Build history of the part. All positions in model axes, mm. Face numbers are marked on the shaded views. A direction names the side the tool comes from. Coordinates: 2 decimals unless noted, no trailing zeros. Order: outer loops, then holes, each group sorted by start corner. A loop starts at its lowest first (then second) coordinate and runs counter-clockwise, first axis right, second up. Notation, with made-up numbers: (-24, 32.5) - (29, 32.5) arc R10 ccw to (29, 49.5) - close; hole circle Ø4 at (22, 56.25). An arc over 180 degrees is marked (long way). One line per item, written item: value.
from build123d import *

# Parameters (mm, degrees)
SKETCH1_W           = 50
SKETCH1_H           = 80
BOSS_EXTRUDE1_DEPTH = 3
SKETCH2_W           = 50
SKETCH2_H           = 3
BOSS_EXTRUDE2_DEPTH = 20
FILLET1_R           = 3
FILLET2_R           = 15
CUT_EXTRUDE1_DEPTH  = 4
CUT_EXTRUDE2_DEPTH  = 81


with BuildPart() as part:
    # Sketch1 → Boss-Extrude1 (new body)
    with BuildSketch(Plane(origin=(0, 0, 0), x_dir=(1, 0, 0), z_dir=(0, 1, 0))):
        Rectangle(SKETCH1_W, SKETCH1_H)
    extrude(amount=BOSS_EXTRUDE1_DEPTH)

    # Sketch2 → Boss-Extrude2 (add)
    with BuildSketch(Plane(origin=(0, 3, 0), x_dir=(1, 0, 0), z_dir=(0, 1, 0))):
        with Locations((0, -38.5)):
            Rectangle(SKETCH2_W, SKETCH2_H)
    extrude(amount=BOSS_EXTRUDE2_DEPTH)

    # Fillet1
    fillet1_edges = [part.edges().sort_by_distance(p)[0] for p in [
        (-25, 23, 38.5),
        (25, 23, 38.5),
    ]]
    fillet(fillet1_edges, radius=FILLET1_R)

    # Fillet2
    fillet2_edges = [part.edges().sort_by_distance(p)[0] for p in [
        (-25, 1.5, -40),
        (25, 1.5, -40),
    ]]
    fillet(fillet2_edges, radius=FILLET2_R)

    # Sketch3 → Cut-Extrude1 (cut, through all)
    with BuildSketch(Plane(origin=(0, 3, 0), x_dir=(1, 0, 0), z_dir=(0, 1, 0))):
        with BuildLine():
            Line((-12.1, 30.1), (12.1, 30.1))
            ThreePointArc((12.1, 30.1), (14.221320344, 29.221320344), (15.1, 27.1))
            Line((15.1, 27.1), (15.1, -27.1))
            ThreePointArc((15.1, -27.1), (14.221320344, -29.221320344), (12.1, -30.1))
            Line((12.1, -30.1), (-12.1, -30.1))
            ThreePointArc((-12.1, -30.1), (-14.221320344, -29.221320344), (-15.1, -27.1))
            Line((-15.1, -27.1), (-15.1, 27.1))
            ThreePointArc((-15.1, 27.1), (-14.221320344, 29.221320344), (-12.1, 30.1))
        make_face()
    extrude(amount=-CUT_EXTRUDE1_DEPTH, mode=Mode.SUBTRACT)

    # Sketch4 → Cut-Extrude2 (cut, through all)
    with BuildSketch(Plane.XY.offset(40)):
        with BuildLine():
            Line((-15, 8.5), (-15, 10))
            Line((-15, 10), (-13.5, 10))
            ThreePointArc((-13.5, 10), (-16.060660172, 11.060660172), (-15, 8.5))
        make_face()
        with BuildLine():
            Line((-13.5, 10), (-15, 10))
            Line((-15, 10), (-15, 8.5))
            ThreePointArc((-15, 8.5), (-13.939339828, 8.939339828), (-13.5, 10))
        make_face()
        with BuildLine():
            ThreePointArc((16.5, 10), (15, 11.5), (13.5, 10))
            Line((13.5, 10), (15, 10))
            Line((15, 10), (15, 8.5))
            ThreePointArc((15, 8.5), (16.060660172, 8.939339828), (16.5, 10))
        make_face()
        with BuildLine():
            Line((15, 10), (13.5, 10))
            ThreePointArc((13.5, 10), (13.939339828, 8.939339828), (15, 8.5))
            Line((15, 8.5), (15, 10))
        make_face()
    extrude(amount=-CUT_EXTRUDE2_DEPTH, mode=Mode.SUBTRACT)


solid = part.part
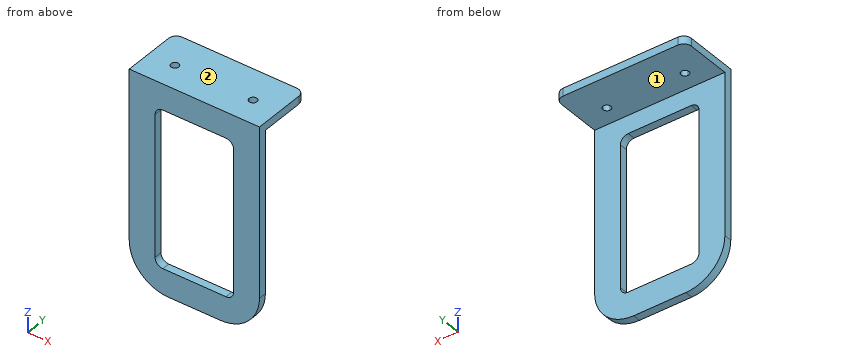
1. Flat gauge pins, fed straight in: P1, Ø1.8, axis at x = -15, y = 10, coming from the +Z side; P2, Ø10, axis at y = 4, z = 28, coming from the +X side. Where does each tip first touch, or does it go through?
Values found:
P1: passes through
P2: stops at x = 25
2. Band-saw the part on B-B, the plane x = -8.5. Give the cut face in (y, z).
Values found:
outline: (0, -40) - (3, -40) - (3, -30.1) - (0, -30.1) - close; (0, 30.1) - (3, 30.1) - (3, 37) - (23, 37) - (23, 40) - (0, 40) - close
3. Band-saw the part on A-A, the plane z = -16.5. Give the cut face in (x, y), and give its area (3 significant figures).
Values found:
outline: (-25, 0) - (-15.1, 0) - (-15.1, 3) - (-25, 3) - close; (15.1, 0) - (25, 0) - (25, 3) - (15.1, 3) - close
area: 59.4 mm2
4. Band-saw the part on C-C, the plane z = -34. Give the cut face in (x, y).
Values found:
outline: (-22, 0) - (22, 0) - (22, 3) - (-22, 3) - close
5. Band-saw the part on D-D, the plane y = 14. Give the cut face in (x, z), and give its area (3 significant figures).
Values found:
outline: (-25, 37) - (25, 37) - (25, 40) - (-25, 40) - close
area: 150 mm2
6. Probe line 1 along X through (y, z) = (10, 38); line 2 along Y through (x, z) = (-15, 38); line 3 along X through (y, z) = (2.25, -23). List the from-to ranges inside material, lowest first.
Values found:
line 1: x = -25 to -16.5, -13.5 to 13.5, 16.5 to 25
line 2: y = 0 to 8.5, 11.5 to 23
line 3: x = -25 to -15.1, 15.1 to 25
7. 3-axis set-ups, long thin cutter, end or side, ignore diameter. For the marked faces 1 and 2: which of +Z, -Z, +X, -X, +Y, -Y reach the whole face in a straight line?
Values found:
face 1: -Z, +X, -X, +Y
face 2: +Z, +X, -X, +Y, -Y
